```python
from build123d import *

# Parameters (mm, degrees)
F3_DEPTH = 66.548


# Not quite as in the source:
# - a feature names something its author has since deleted; it is built from what else it names


with BuildPart() as f1:
    # F0 (on Right) → F1 (revolve)
    with BuildSketch(Plane.YZ):
        Polygon((-107.315, 14.605), (-135.1026, 14.605), (-135.1026, 0), (0, 0), (293.1414, 0), (293.1414, 17.4625), (192.0494, 17.4625), (192.0494, 18.2626), (161.5948, 18.2626), (161.5948, 20.6375), (-69.088, 20.6375), (-69.088, 18.2626), (-72.39, 18.2626), (-72.39, 14.9606), (-107.315, 14.9606), align=None)
    revolve(axis=Axis((0, 146.5707, 0), (0, -1, 0)))

    # F2 (on face) → F3 (cut)
    with BuildSketch(Plane(origin=(0, 293.1414, 0), x_dir=(-1, 0, 0), z_dir=(0, 1, 0))):
        with BuildLine():
            Line((-3.96875, 17.0055264455), (-3.96875, 12.8397))
            Line((-3.96875, 12.8397), (3.96875, 12.8397))
            Line((3.96875, 12.8397), (3.96875, 17.0055264455))
            ThreePointArc((3.96875, 17.0055264455), (0, 17.4625), (-3.96875, 17.0055264455))
        make_face()
    extrude(amount=-F3_DEPTH, mode=Mode.SUBTRACT)


solid = f1.part
```
Could you check a few things on this model? Use its own coordinates, in mm. A direction names the side the tool comes from. Give positions to 0.01 mm unless a question says otherwise; leave off trailing zeros. Order: outer loops, then holes, each group sorted by start corner. A loop starts at its lowest first (then second) coordinate and runs counter-clockwise, first axis right, second up.
Q1. I'm going to push flat-ended pins straight in: P1, Ø10, axis at y = 145.5, z = 5.5, coming from the -X side; P2, Ø6, axis at x = -11, y = 233.5, coming from the +Z side; P3, Ø3.5, axis at x = 2, z = 16, coming from the +Y side. Where does each tip first touch, or does it pass through?
Q2. Suppose I cut it at C-C, the plane y = 8. Write out the boundary of the cut face in (x, z) (1 decimal), and give its area (3 significant figures).
Q3. We'd pull the mould along X, two halves only. Please class faces 1 (the flat face through (0, 260, 12.84)), 2 (the cylindrical face through (20.147, 44.639, -4.474)), 3 (the flat face through (7, -107.315, 13)): +X half, -X half, draft (parallel to the pull), parting line (faces both ways), or undercut.
Q4. Suppose I cut it at D-D, the plane y = 262. Write out the boundary of the cut face in (x, z) (1 decimal), and give its area (3 significant figures).
Q5. If I drill on line 1 along Y through (x, z) = (6, 18.5); line 2 along X through (y, z) = (-71, 5.5); line 3 along Y through (x, z) = (12.5, -11), over which ranges is the centre line in solid material (lowest first)?
Q6. For faces 4 (the flat face through (0, 293.141, 0)), 5 (the cylindrical face through (-5.486, -70.762, 17.419)), 6 (the cylindrical face through (-5.486, 176.609, 17.419)), which set-ups out of +Z, -Z, +X, -X, +Y, -Y let a thin tool reach every point of the face, with its end or its side?
Solution:
1. P1: stops at x = -20.63
1. P2: stops at z = 15.52
1. P3: stops at y = 226.59
2. outline: circle Ø41.3 at (0, 0)
2. area: 1,340 mm2
3. face 1: undercut
3. face 2: parting line
3. face 3: draft
4. outline: (-4, 12.8) - (-4, 17) arc R17.5 ccw (long way) to (4, 17) - (4, 12.8) - close
4. area: 923 mm2
5. line 1: y = -69.09 to 161.59
5. line 2: x = -17.41 to 17.41
5. line 3: y = -72.39 to 293.14
6. face 4: +Z, -Z, +X, -X, +Y
6. face 5: -Y
6. face 6: +Y
